For this review, take the finished solid that the model builds, in its own axes (mm). A direction names the side the tool comes from. Coordinates: 2 decimals unless noted, no trailing zeros. Write each loop counter-clockwise with the first axis right and the second up, starting at its lowest first coordinate (ties: lowest second). Pieces come first, ordered by that corner, then holes. Notation, with made-up numbers: (69.5, 55) - (122.5, 55) arc R6 ccw to (122.5, 63) - close; hole circle Ø4 at (40.5, 40.5). An arc over 180 degrees is marked (long way). Use one line per item in the form item = value. Start each with the question number.
1) We need section B-B (z = 9). Give the boundary of the cut face in (x, y), plus the area to 3 significant figures.
2) For L1, parallel to Y at x = -25, z = 3; L2, parallel to Z at x = 25, y = 1.9 (3 decimals); L3, parallel to X at y = 2, z = 47, list the stretches that pass through material, from the lowest coordinate up. Write a range as from..to.
3) We need section A-A (x = 25). Give the boundary of the cut face in (y, z) (3 decimals).
4) Mouldability with a two-part tool opening along Y and no side actions: class faces 1 (the flat face through (17.5, 24, 28)), 2 (the flat face through (-0.245, 27.308, 29.157)), 3 (the cylindrical face through (-23.777, 12.649, 2.535)) as pulls with the +Y half, pulls with the -Y half, needs draft (parallel to the pull), parting line crosses it, or undercut.
5) We need section C-C (y = 15). Give the boundary of the cut face in (x, z), plus the area to 3 significant figures.
6) Tool access review of faces 4 (the flat face through (20, 2, 25)), 5 (the flat face through (0, 2, 45)), 6 (the flat face through (0, 25, 0)): name each direction out of +Z, -Z, +X, -X, +Y, -Y from which nothing blocks a thin tool from reaching the whole face with its end or side.
7) We need section D-D (x = 0.5). Give the boundary of the cut face in (y, z).
8) Insertion check: P1, Ø5.5, axis at x = -4, y = 2.5, coming from the -Z side; P2, Ø6, axis at y = 14.5, z = 43, coming from the +X side; P3, Ø4, axis at x = 25, z = 47.5, coming from the -Y side; P4, Ø8, axis at y = 42.5, z = 11, coming from the -X side. Each pin has a flat end and moves straight along its axis. Give the tip position at first contact, or say it passes through.
```python
from build123d import *

# Parameters (mm, degrees)
SKETCH1_W           = 65
SKETCH1_H           = 50
BOSS_EXTRUDE1_DEPTH = 5
SKETCH7_W           = 65
SKETCH7_H           = 50
BOSS_EXTRUDE5_DEPTH = 50
CUT_EXTRUDE4_DEPTH  = 99.742088291
SKETCH9_R           = 2.65
CUT_EXTRUDE5_DEPTH  = 78.821912081
SKETCH10_R          = 3.125
CUT_EXTRUDE6_DEPTH  = 79.14249804
CUT_EXTRUDE14_DEPTH = 15
CUT_EXTRUDE15_START = -65
CUT_EXTRUDE15_DEPTH = 15
CUT_EXTRUDE16_DEPTH = 99.742088291
CUT_EXTRUDE17_REACH = 83.125
SKETCH26_W          = 40
SKETCH26_H          = 40


with BuildPart() as part:
    # Sketch1 → Boss-Extrude1 (new body)
    with BuildSketch(Plane.XY):
        with Locations((0, 25)):
            Rectangle(SKETCH1_W, SKETCH1_H)
    extrude(amount=BOSS_EXTRUDE1_DEPTH)

    # Sketch7 → Boss-Extrude5 (add)
    with BuildSketch(Plane.XY.offset(5)):
        with Locations((0, 25)):
            Rectangle(SKETCH7_W, SKETCH7_H)
    extrude(amount=BOSS_EXTRUDE5_DEPTH)

    # Sketch8 → Cut-Extrude4 (cut, through all)
    with BuildSketch(Plane.ZY.offset(32.5)):
        Polygon((55, 50), (5, 50), (5, 49), (54, 5), (55, 5), align=None)
    extrude(amount=-CUT_EXTRUDE4_DEPTH, mode=Mode.SUBTRACT)

    # Sketch9 → Cut-Extrude5 (cut, through all)
    with BuildSketch(Plane.XY.offset(5)):
        with Locations((-25, 15)):
            Circle(SKETCH9_R)
        with Locations(Location((25, 15, 0), (0, 0, 180))):
            Circle(SKETCH9_R)
    extrude(amount=-CUT_EXTRUDE5_DEPTH, mode=Mode.SUBTRACT)

    # Sketch10 → Cut-Extrude6 (cut, through all)
    with BuildSketch(Plane(origin=(0, 5, 0), x_dir=(1, 0, 0), z_dir=(0, 1, 0))):
        with Locations(Location((-25, -47.5, 0), (0, 0, 180))):
            Circle(SKETCH10_R)
        with Locations((25, -47.5)):
            Circle(SKETCH10_R)
    extrude(amount=-CUT_EXTRUDE6_DEPTH, mode=Mode.SUBTRACT)

    # Sketch24 → Cut-Extrude14 (cut)
    with BuildSketch(Plane(origin=(32.5, 0, 0), x_dir=(0, 0, -1), z_dir=(1, 0, 0))):
        Polygon((-5, 49), (-54, 5), (-5, 5), align=None)
    extrude(amount=-CUT_EXTRUDE14_DEPTH, mode=Mode.SUBTRACT)

    # Sketch24<2> → Cut-Extrude15 (cut)
    with BuildSketch(Plane(origin=(32.5, 0, 0), x_dir=(0, 0, -1), z_dir=(1, 0, 0)).offset(CUT_EXTRUDE15_START)):
        Polygon((-5, 49), (-54, 5), (-5, 5), align=None)
    extrude(amount=CUT_EXTRUDE15_DEPTH, mode=Mode.SUBTRACT)

    # Sketch25 → Cut-Extrude16 (cut, through all)
    with BuildSketch(Plane(origin=(32.5, 0, 0), x_dir=(0, 0, -1), z_dir=(1, 0, 0))):
        Polygon((-5, 5), (-5, 42.280009867), (-46.516374625, 5), align=None)
    extrude(amount=-CUT_EXTRUDE16_DEPTH, mode=Mode.SUBTRACT)

    # Sketch26 → Cut-Extrude17 (cut, up to next)
    with BuildSketch(Plane.XZ, mode=Mode.PRIVATE) as cut_extrude17_sk1:
        with Locations((0, 25)):
            Rectangle(SKETCH26_W, SKETCH26_H)
    cut_extrude17_tool1 = extrude(cut_extrude17_sk1.sketch, amount=-CUT_EXTRUDE17_REACH, mode=Mode.PRIVATE) & part.part
    add(cut_extrude17_tool1.solids().sort_by_distance((0, 0, 25))[0], mode=Mode.SUBTRACT)


solid = part.part
```
Determined:
q1.outline = (-32.5, 0) - (-20, 0) - (-20, 5) - (-32.5, 5) - close; (-17.5, 38.69) - (17.5, 38.69) - (17.5, 45.41) - (-17.5, 45.41) - close; (20, 0) - (32.5, 0) - (32.5, 5) - (20, 5) - close
q1.area = 360 mm²
q2.L1 = 0..12.35, 17.65..50
q2.L2 = 0..44.375, 50.625..55
q2.L3 = -32.5..-28.08, -21.92..21.92, 28.08..32.5
q3.outline = (0, 0) - (12.35, 0) - (12.35, 5) - (5, 5) - (5, 44.375) - (0, 44.375) - close; (0, 50.625) - (5, 50.625) - (5, 55) - (0, 55) - close; (17.65, 0) - (50, 0) - (50, 5) - (17.65, 5) - close
q4.face_1 = needs draft
q4.face_2 = pulls with the +Y half
q4.face_3 = undercut
q5.outline = (-32.5, 0) - (-27.65, 0) - (-27.65, 5) - (-32.5, 5) - close; (-22.35, 0) - (22.35, 0) - (22.35, 5) - (-22.35, 5) - close; (-17.5, 35.38) - (17.5, 35.38) - (17.5, 42.86) - (-17.5, 42.86) - close; (27.65, 0) - (32.5, 0) - (32.5, 5) - (27.65, 5) - close
q5.area = 534 mm²
q6.face_4 = +Y, -Y
q6.face_5 = -Y
q6.face_6 = -Z, +X, -X, +Y, -Y
q7.outline = (0, 0) - (50, 0) - (50, 5) - (49, 5) - (5, 54) - (5, 55) - (0, 55) - (0, 45) - (5, 45) - (5, 46.52) - (42.28, 5) - (0, 5) - close
q8.P1 = 0
q8.P2 = 17.5
q8.P3 = through
q8.P4 = -17.5
